Geometry check sheet. Reference: the model listing, model coordinates, mm. Face numbers are marked on the shaded views. Round coordinates to 2 decimals unless told otherwise and drop trailing zeros. Order: outer loops, then holes, each group sorted by start corner. A loop starts at its lowest first (then second) coordinate and runs counter-clockwise, first axis right, second up.
```python
from build123d import *

# Parameters (mm, degrees)
P_IDAT_VYSUNUT_M2_DEPTH  = 2.5
SKICA3_W                 = 0.8
SKICA3_H                 = 0.8
ODEBRAT_VYSUNUT_M1_DEPTH = 2.5
SKICA4_W                 = 8.539651134
SKICA4_H                 = 7.495504433
ODEBRAT_VYSUNUT_M2_DEPTH = 2.5


# Read off the part's stored shape, not the designer's step: Přidat vysunutím2
with BuildPart() as part:
    # Přidat vysunutím2 outline → Přidat vysunutím2 (new body)
    with BuildSketch(Plane.XY):
        with BuildLine():
            Line((2.40336004, -19.590083306), (2.40336004, -16.441317707))
            ThreePointArc((2.40336004, -16.441317707), (1.30336004, -15.341317707), (0.20336004, -16.441317707))
            Line((0.20336004, -16.441317707), (-0.14663996, -16.441317707))
            ThreePointArc((-0.14663996, -16.441317707), (-1.24602276, -15.34131788), (-2.346639267, -16.440083307))
            Line((-2.346639267, -16.440083307), (-2.696640653, -16.440083307))
            ThreePointArc((-2.696640653, -16.440083307), (-3.79725716, -15.34131788), (-4.89663996, -16.441317707))
            Line((-4.89663996, -16.441317707), (-5.24663996, -16.441317707))
            ThreePointArc((-5.24663996, -16.441317707), (-6.34663996, -15.341317707), (-7.44663996, -16.441317707))
            Line((-7.44663996, -16.441317707), (-7.79663996, -16.441317707))
            Line((-7.79663996, -16.441317707), (-7.79663996, -16.399925636))
            ThreePointArc((-7.79663996, -16.399925636), (-8.89663996, -15.299925636), (-9.99663996, -16.399925636))
            Line((-9.99663996, -16.399925636), (-9.99663996, -16.441317707))
            Line((-9.99663996, -16.441317707), (-10.34663996, -16.441317707))
            ThreePointArc((-10.34663996, -16.441317707), (-11.44663996, -15.341317707), (-12.54663996, -16.441317707))
            Line((-12.54663996, -16.441317707), (-12.89663996, -16.441317707))
            ThreePointArc((-12.89663996, -16.441317707), (-13.99663996, -15.341317707), (-15.09663996, -16.441317707))
            Line((-15.09663996, -16.441317707), (-15.09663996, -19.590083306))
            ThreePointArc((-15.09663996, -19.590083306), (-13.99663996, -20.690083306), (-12.89663996, -19.590083306))
            Line((-12.89663996, -19.590083306), (-12.54663996, -19.590083306))
            ThreePointArc((-12.54663996, -19.590083306), (-11.44663996, -20.690083306), (-10.34663996, -19.590083306))
            Line((-10.34663996, -19.590083306), (-9.99663996, -19.590083306))
            Line((-9.99663996, -19.590083306), (-9.99663996, -19.631475378))
            ThreePointArc((-9.99663996, -19.631475378), (-8.89663996, -20.731475378), (-7.79663996, -19.631475378))
            Line((-7.79663996, -19.631475378), (-7.79663996, -19.590083306))
            Line((-7.79663996, -19.590083306), (-7.44663996, -19.590083306))
            ThreePointArc((-7.44663996, -19.590083306), (-6.34663996, -20.690083306), (-5.24663996, -19.590083306))
            Line((-5.24663996, -19.590083306), (-4.89663996, -19.590083306))
            ThreePointArc((-4.89663996, -19.590083306), (-3.79663996, -20.690083306), (-2.69663996, -19.590083306))
            Line((-2.69663996, -19.590083306), (-2.34663996, -19.590083306))
            ThreePointArc((-2.34663996, -19.590083306), (-1.24663996, -20.690083306), (-0.14663996, -19.590083306))
            Line((-0.14663996, -19.590083306), (0.20336004, -19.590083306))
            ThreePointArc((0.20336004, -19.590083306), (1.30336004, -20.690083306), (2.40336004, -19.590083306))
        make_face()
    extrude(amount=P_IDAT_VYSUNUT_M2_DEPTH)

    # Skica3 → Odebrat vysunutím1 (cut)
    with BuildSketch(Plane.XY.offset(2.5)):
        with Locations((-13.99663996, -16.715700507)):
            Rectangle(SKICA3_W, SKICA3_H)
        with Locations((-13.99663996, -19.315700507)):
            Rectangle(SKICA3_W, SKICA3_H)
        with Locations((-8.89663996, -16.715700507)):
            Rectangle(SKICA3_W, SKICA3_H)
        with Locations((-11.44663996, -16.715700507)):
            Rectangle(SKICA3_W, SKICA3_H)
        with Locations((-11.44663996, -19.315700507)):
            Rectangle(SKICA3_W, SKICA3_H)
        with Locations((-8.89663996, -19.315700507)):
            Rectangle(SKICA3_W, SKICA3_H)
        with Locations((-6.34663996, -16.715700507)):
            Rectangle(SKICA3_W, SKICA3_H)
        with Locations((-6.34663996, -19.315700507)):
            Rectangle(SKICA3_W, SKICA3_H)
        with Locations((-3.79663996, -16.715700507)):
            Rectangle(SKICA3_W, SKICA3_H)
        with Locations((-3.79663996, -19.315700507)):
            Rectangle(SKICA3_W, SKICA3_H)
        with Locations((-1.24663996, -16.715700507)):
            Rectangle(SKICA3_W, SKICA3_H)
        with Locations((-1.24663996, -19.315700507)):
            Rectangle(SKICA3_W, SKICA3_H)
        with Locations((1.30336004, -16.715700507)):
            Rectangle(SKICA3_W, SKICA3_H)
        with Locations((1.30336004, -19.315700507)):
            Rectangle(SKICA3_W, SKICA3_H)
    extrude(amount=-ODEBRAT_VYSUNUT_M1_DEPTH, mode=Mode.SUBTRACT)

    # Skica4 → Odebrat vysunutím2 (cut)
    with BuildSketch(Plane.XY.offset(2.5)):
        with Locations((-0.976814393, -18.745431106)):
            Rectangle(SKICA4_W, SKICA4_H)
    extrude(amount=-ODEBRAT_VYSUNUT_M2_DEPTH, mode=Mode.SUBTRACT)


solid = part.part
```
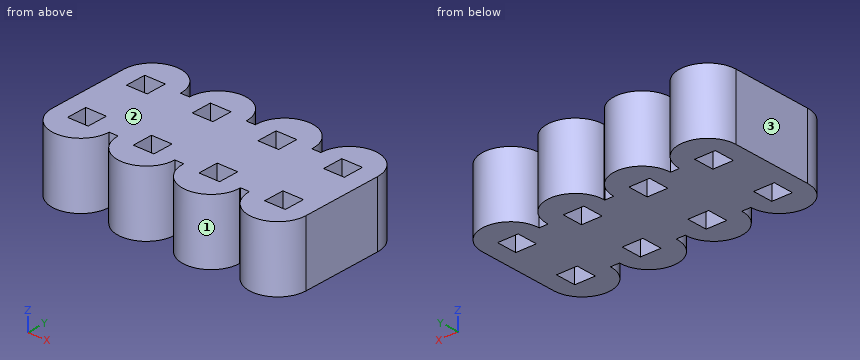
(1) Sectioned sample at C-C, the plane z = 0.7. Give the number of separate pieces and of enclosed holes in the cut face, and give its area (3 significant figures).
Returned:
separate pieces: 1
enclosed holes: 8
area: 41.3 mm2
(2) Material ranges on line 1 (X direction, y = -19.35, z = 1.1); line 2 (X direction, y = -15.75, z = 1.8); line 3 (X direction, y = -15.6, z = 0.4), recorded low to high.
Returned:
line 1: x = -15.1 to -14.4, -13.6 to -11.85, -11.05 to -9.3, -8.5 to -6.75, -5.95 to -5.25
line 2: x = -14.85 to -13.14, -12.3 to -10.59, -9.78 to -8.01, -7.2 to -5.49
line 3: x = -14.71 to -13.29, -12.16 to -10.74, -9.65 to -8.14, -7.06 to -5.64
(3) Sectioned sample at B-B, the plane x = -6.5. Record the cut outline in (y, z).
Returned:
outline: (-20.68, 0) - (-19.72, 0) - (-19.72, 2.5) - (-20.68, 2.5) - close; (-18.92, 0) - (-17.12, 0) - (-17.12, 2.5) - (-18.92, 2.5) - close; (-16.32, 0) - (-15.35, 0) - (-15.35, 2.5) - (-16.32, 2.5) - close
(4) Draft check along X on the marked faces 1, 2 and 3. Enter one of: released by +X, released by -X, zero draft, split by the parting line, or undercut.
Returned:
face 1: undercut
face 2: zero draft
face 3: released by -X
(5) Sectioned sample at D-D, the plane y = -20.15. Record the cut outline in (x, z).
Returned:
outline: (-14.94, 0) - (-13.05, 0) - (-13.05, 2.5) - (-14.94, 2.5) - close; (-12.39, 0) - (-10.5, 0) - (-10.5, 2.5) - (-12.39, 2.5) - close; (-9.87, 0) - (-7.93, 0) - (-7.93, 2.5) - (-9.87, 2.5) - close; (-7.29, 0) - (-5.4, 0) - (-5.4, 2.5) - (-7.29, 2.5) - close
(6) Sectioned sample at A-A, the plane y = -15.95. Record the cut outline in (x, z), and give its area (3 significant figures).
Returned:
outline: (-14.98, 0) - (-13.01, 0) - (-13.01, 2.5) - (-14.98, 2.5) - close; (-12.43, 0) - (-10.46, 0) - (-10.46, 2.5) - (-12.43, 2.5) - close; (-9.9, 0) - (-7.89, 0) - (-7.89, 2.5) - (-9.9, 2.5) - close; (-7.33, 0) - (-5.36, 0) - (-5.36, 2.5) - (-7.33, 2.5) - close
area: 19.8 mm2
(7) Depth check by flat-ended pin: P1, Ø0.6, axis at x = -14, z = 1.5, coming from the -Y side; P2, Ø1, axis at x = -6.5, z = 0.5, coming from the +Y side. Enter the tip coordinate at first touch or a pass-through.
Returned:
P1: stops at y = -20.69
P2: stops at y = -15.34
